Part model, mm, in its own coordinate system. A direction names the side the tool comes from. Give positions to 0.01 mm unless a question says otherwise; leave off trailing zeros. Write each loop counter-clockwise with the first axis right and the second up, starting at its lowest first coordinate (ties: lowest second). Pieces come first, ordered by that corner, then holes.
from build123d import *
from OCP.BRepFilletAPI import BRepFilletAPI_MakeFillet

# Parameters (mm, degrees)
SKETCH1_R           = 4.5
SKETCH1_R_2         = 3.302
BOSS_EXTRUDE1_DEPTH = 6.35
FILLET2_R           = 7.5
FILLET2_R_2         = 3.5


with BuildPart() as part:
    # Sketch1 → Boss-Extrude1 (new body)
    with BuildSketch(Plane.XY):
        Polygon((0, 0), (37.6, 0), (37.6, 25.4), (26.3, 25.4), (26.3, 37.4), (11.3, 37.4), (11.3, 25.4), (0, 25.4), align=None)
        with Locations((18.8, 29.9)):
            Circle(SKETCH1_R, mode=Mode.SUBTRACT)
        with Locations((6.3, 12.7)):
            Circle(SKETCH1_R_2, mode=Mode.SUBTRACT)
        with Locations((31.3, 12.7)):
            Circle(SKETCH1_R_2, mode=Mode.SUBTRACT)
    extrude(amount=BOSS_EXTRUDE1_DEPTH)

    # Fillet2
    fillet2_edges_1 = [part.edges().sort_by_distance(p)[0] for p in [
        (11.3, 37.4, 3.175),
        (26.3, 37.4, 3.175),
    ]]
    fillet2_edges_2 = [part.edges().sort_by_distance(p)[0] for p in [
        (11.3, 25.4, 3.175),
        (0, 25.4, 3.175),
        (0, 0, 3.175),
        (37.6, 25.4, 3.175),
        (26.3, 25.4, 3.175),
        (37.6, 0, 3.175),
    ]]
    fillet2 = BRepFilletAPI_MakeFillet(part.part.solid().wrapped)
    for e in fillet2_edges_1:
        fillet2.Add(FILLET2_R - 0.0001, e.wrapped)
    for e in fillet2_edges_2:
        fillet2.Add(FILLET2_R_2 - 0.0001, e.wrapped)
    add(Compound.cast(fillet2.Shape()), mode=Mode.REPLACE)  # a hair under: the kernel refuses the full size


solid = part.part
1) Drill centre lines: L1, parallel to Y at x = 31.3, z = 3.5; L2, parallel to Y at x = 18.8, z = 1.5; L3, parallel to X at y = 11, z = 4. Where is each one in solid material? Low to high.
Check result:
L1: y = 0 to 9.4, 16 to 25.4
L2: y = 0 to 25.4, 34.4 to 37.4
L3: x = 0 to 3.47, 9.13 to 28.47, 34.13 to 37.6
2) Saw through at D-D (y = 26.5). Write the cut outline in (x, z), and give its area (3 significant figures).
Check result:
outline: (10.35, 0) - (15.85, 0) - (15.85, 6.35) - (10.35, 6.35) - close; (21.75, 0) - (27.25, 0) - (27.25, 6.35) - (21.75, 6.35) - close
area: 69.9 mm2
3) 3-axis set-ups, long thin cutter, end or side, ignore diameter. For faces 4 (the flat face through (6, 25.4, 3)), 5 (the flat face through (0, 13, 3)), 6 (the flat face through (32, 25.4, 3)): which of +Z, -Z, +X, -X, +Y, -Y reach the whole face in a straight line?
Check result:
face 4: +Z, -Z, -X, +Y
face 5: +Z, -Z, -X, +Y, -Y
face 6: +Z, -Z, +X, +Y
4) Saw through at B-B (z = 3). State how many separate pieces and enclosed holes the cut face has, and give its area (3 significant figures).
Check result:
separate pieces: 1
enclosed holes: 3
area: 974 mm2
5) Saw through at C-C (x = 31.3). Write the cut outline in (y, z), and give its area (3 significant figures).
Check result:
outline: (0, 0) - (9.4, 0) - (9.4, 6.35) - (0, 6.35) - close; (16, 0) - (25.4, 0) - (25.4, 6.35) - (16, 6.35) - close
area: 119 mm2
6) Flat gauge pins, fed straight in: P1, Ø1.5, axis at x = 33, z = 2, coming from the +Y side; P2, Ø0.5, axis at y = 29.5, z = 3.5, coming from the -X side. Where does each tip first touch, or does it go through?
Check result:
P1: stops at y = 25.4
P2: stops at x = 11.3
7) Saw through at A-A (y = 12.7). Write the cut outline in (x, z).
Check result:
outline: (0, 0) - (3, 0) - (3, 6.35) - (0, 6.35) - close; (9.6, 0) - (28, 0) - (28, 6.35) - (9.6, 6.35) - close; (34.6, 0) - (37.6, 0) - (37.6, 6.35) - (34.6, 6.35) - close
8) Mould opens along X. For faces 1 (the cylindrical face through (13.439, 35.145, 3.219)), 2 (the cylindrical face through (28.866, 14.932, 3.131)), 3 (the flat face through (26.3, 29.4, 3.1)) say: +X half, -X half, draft (parallel to the pull), parting line (faces both ways), or undercut.
Check result:
face 1: -X half
face 2: undercut
face 3: +X half
